Geometry: final body of the model. Coordinates: model frame, mm. Give positions to 0.01 mm unless a question says otherwise; leave off trailing zeros. Write each loop counter-clockwise with the first axis right and the second up, starting at its lowest first coordinate (ties: lowest second). Pieces come first, ordered by that corner, then holes. Notation, with made-up numbers: M -7,59 L 32,59 A3 cw 32,64 Z; hole C 53.25,-31 d8. An arc over 180 degrees is marked long. Use a Markdown table: item, result. Add a question column.
1) Section A-A on x = -0.5. Return the cut outline in (y, z), then the cut area to 3 significant figures.
2) Line query: line 1 (Y direction, x = -0.25, z = 13.5); line 2 (X direction, y = 5.5, z = 4); line 3 (X direction, y = -4.25, z = 12.5). Output: solid intervals per line, ascending.
3) Section B-B on z = 10.5. Return the cut outline in (x, y).
```python
from build123d import *

# Parameters (mm, degrees)
F1_DEPTH = 15.24
F2_R     = 3.81


with BuildPart() as f1:
    # F0 (on Top) → F1 (new body)
    with BuildSketch(Plane.XY):
        with BuildLine():
            Line((-3.81, -7.62), (3.81, -7.62))
            ThreePointArc((3.81, -7.62), (6.5040768363, -6.5040768363), (7.62, -3.81))
            Line((7.62, -3.81), (7.62, 3.81))
            ThreePointArc((7.62, 3.81), (6.5040768363, 6.5040768363), (3.81, 7.62))
            Line((3.81, 7.62), (-3.81, 7.62))
            ThreePointArc((-3.81, 7.62), (-6.5040768363, 6.5040768363), (-7.62, 3.81))
            Line((-7.62, 3.81), (-7.62, -3.81))
            ThreePointArc((-7.62, -3.81), (-6.5040768363, -6.5040768363), (-3.81, -7.62))
        make_face()
    extrude(amount=F1_DEPTH)

    # F2
    f2_edges = [f1.edges().sort_by_distance(p)[0] for p in [
        (-7.62, 0, 15.24),
        (-6.504077, -6.504077, 15.24),
        (0, -7.62, 15.24),
        (6.504077, -6.504077, 15.24),
        (7.62, 0, 15.24),
        (6.504077, 6.504077, 15.24),
        (0, 7.62, 15.24),
        (-6.504077, 6.504077, 15.24),
        (-7.62, 0, 0),
        (-6.504077, -6.504077, 0),
        (0, -7.62, 0),
        (6.504077, -6.504077, 0),
        (7.62, 0, 0),
        (6.504077, 6.504077, 0),
        (0, 7.62, 0),
        (-6.504077, 6.504077, 0),
    ]]
    fillet(f2_edges, radius=F2_R)


solid = f1.part
```
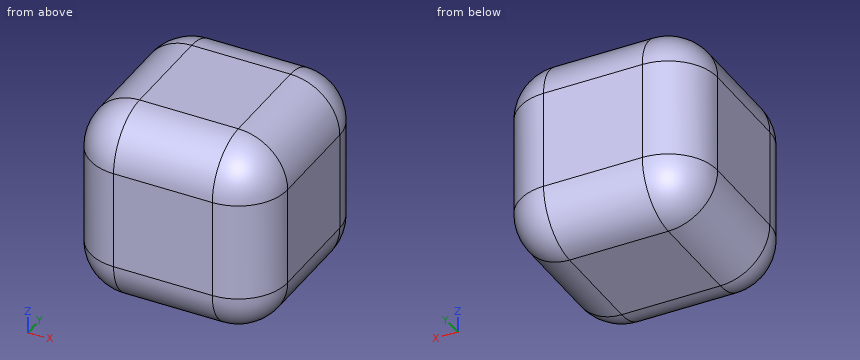
Found:
| question | item | result |
|---|---|---|
| 1 | outline | M -7.62,3.81 A3.81 ccw -3.81,0 L 3.81,0 A3.81 ccw 7.62,3.81 L 7.62,11.43 A3.81 ccw 3.81,15.24 L -3.81,15.24 A3.81 ccw -7.62,11.43 Z |
| 1 | area | 220 mm² |
| 2 | line 1 | -7.01 to 7.01 |
| 2 | line 2 | -7.22 to 7.22 |
| 2 | line 3 | -7.44 to 7.44 |
| 3 | outline | M -7.62,-3.81 A3.81 ccw -3.81,-7.62 L 3.81,-7.62 A3.81 ccw 7.62,-3.81 L 7.62,3.81 A3.81 ccw 3.81,7.62 L -3.81,7.62 A3.81 ccw -7.62,3.81 Z |
